Source: CAD feature listing. Evaluate the final solid. Frame: model axes, mm. Face numbers are marked on the shaded views. A direction names the side the tool comes from. Give positions to 0.01 mm unless a question says otherwise; leave off trailing zeros. Order: outer loops, then holes, each group sorted by start corner. A loop starts at its lowest first (then second) coordinate and runs counter-clockwise, first axis right, second up. Notation, with made-up numbers: (-6, -7.75) - (18, -7.75) arc R23 ccw to (18, 16.25) - close; hole circle Ø10 at (-17.75, 24.25). An arc over 180 degrees is marked (long way). Use CSV: the item, a comma, the result in double quotes.
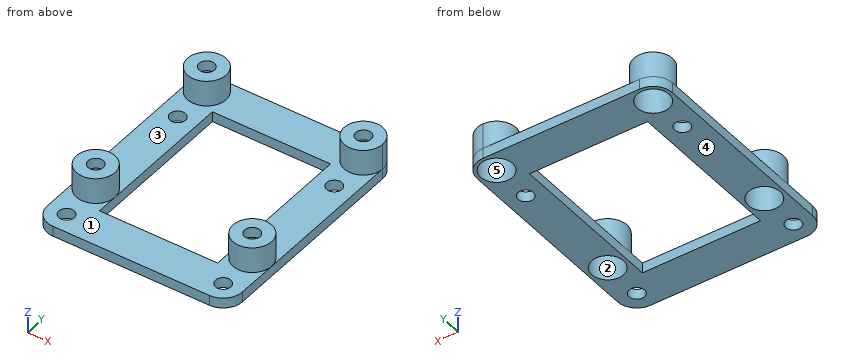
```python
from build123d import *

# Parameters (mm, degrees)
F3_W     = 38
F3_H     = 46
F3_R     = 1.5
F3_W_2   = 23
F3_H_2   = 31
F4_DEPTH = 2
F5_R     = 1.5
F6_DEPTH = 5
F7_R     = 3.7499
F8_R     = 3.1
F9_DEPTH = 5


# Not quite as in the source:
# - a fillet or chamfer is up to 0.001 mm smaller than in the source, because OpenCascade refuses the exact size


with BuildPart() as f4:
    # F3 (on Top) → F4 (new body)
    with BuildSketch(Plane.XY):
        Rectangle(F3_W, F3_H)
        with Locations((-15.25, -19.25)):
            Circle(F3_R, mode=Mode.SUBTRACT)
        with Locations((-15.25, -11.25)):
            Circle(F3_R, mode=Mode.SUBTRACT)
        with Locations((15.25, -19.25)):
            Circle(F3_R, mode=Mode.SUBTRACT)
        with Locations((15.25, -11.25)):
            Circle(F3_R, mode=Mode.SUBTRACT)
        with Locations((-15.25, 11.25)):
            Circle(F3_R, mode=Mode.SUBTRACT)
        with Locations((-15.25, 19.25)):
            Circle(F3_R, mode=Mode.SUBTRACT)
        Rectangle(F3_W_2, F3_H_2, mode=Mode.SUBTRACT)
        with Locations((15.25, 11.25)):
            Circle(F3_R, mode=Mode.SUBTRACT)
        with Locations((15.25, 19.25)):
            Circle(F3_R, mode=Mode.SUBTRACT)
    extrude(amount=F4_DEPTH)

    # F5 (on face) → F6 (join)
    with BuildSketch(Plane.XY.offset(2)):
        with BuildLine():
            ThreePointArc((-19, 19.25), (-15.25, 15.5), (-11.5, 19.25))
            ThreePointArc((-11.5, 19.25), (-12.598349559, 21.9016504179), (-15.2499999673, 23))
            ThreePointArc((-15.2499999673, 23), (-17.9016504179, 21.901650441), (-19, 19.25))
        make_face()
        with Locations((-15.25, 19.25)):
            Circle(F5_R, mode=Mode.SUBTRACT)
        with BuildLine():
            ThreePointArc((19, 19.25), (17.9016504294, 21.9016504294), (15.25, 23))
            ThreePointArc((15.25, 23), (12.5983495706, 16.5983495706), (19, 19.25))
        make_face()
        with Locations((15.25, 19.25)):
            Circle(F5_R, mode=Mode.SUBTRACT)
        with BuildLine():
            ThreePointArc((11.5, -11.25), (15.25, -15), (19, -11.25))
            ThreePointArc((19, -11.25), (15.25, -7.5), (11.5, -11.25))
        make_face()
        with Locations((15.25, -11.25)):
            Circle(F5_R, mode=Mode.SUBTRACT)
        with BuildLine():
            ThreePointArc((-11.5, -11.25), (-15.2499999923, -7.5), (-19, -11.2499999846))
            ThreePointArc((-19, -11.2499999846), (-15.2500000077, -15), (-11.5, -11.25))
        make_face()
        with Locations((-15.25, -11.25)):
            Circle(F5_R, mode=Mode.SUBTRACT)
    extrude(amount=F6_DEPTH)

    # F7 (radius 3.75 in the source; OpenCascade refuses exactly that, so slightly less here)
    f7_edges = [f4.edges().sort_by_distance(p)[0] for p in [
        (-19, 23, 1),
        (-19, -23, 1),
        (19, -23, 1),
        (19, 23, 1),
    ]]
    fillet(f7_edges, radius=F7_R)

    # F8 (on face) → F9 (cut)
    with BuildSketch(Plane(origin=(0, 0, 0), x_dir=(1, 0, 0), z_dir=(0, 0, -1))):
        with Locations((-15.25, 11.25)):
            Circle(F8_R)
        with Locations((15.25, 11.25)):
            Circle(F8_R)
        with Locations((15.25, -19.25)):
            Circle(F8_R)
        with Locations((-15.25, -19.25)):
            Circle(F8_R)
    extrude(amount=-F9_DEPTH, mode=Mode.SUBTRACT)


solid = f4.part
```
Item 1: Section A-A on y = 11.25. Return the cut outline in (x, z), then the cut area to 3 significant figures.
Filled in:
outline,"(-19, 0) - (-16.75, 0) - (-16.75, 2) - (-19, 2) - close; (-13.75, 0) - (-11.5, 0) - (-11.5, 2) - (-13.75, 2) - close; (11.5, 0) - (13.75, 0) - (13.75, 2) - (11.5, 2) - close; (16.75, 0) - (19, 0) - (19, 2) - (16.75, 2) - close"
area,"18.0 mm2"
Item 2: Mould query, pull axis Y, two halves, no side actions, for the marked faces 1 and 2. Classes: released by +Y, released by -Y, zero draft, split by the parting line, or undercut.
Filled in:
face 1,"zero draft"
face 2,"undercut"
Item 3: First-contact query: pin 1 (5 mm diameter, centred on x = -15.25, y = -11.25, fed in from -Z). Flat tip, straight axial feed; report the tip coordinate or a pass-through.
Filled in:
pin 1,"stops at z = 5"
Item 4: Material intervals for line 1 (Y direction, x = 15.25, z = 6); line 2 (X direction, y = 19.25, z = 6.3); line 3 (Y direction, x = 15.25, z = 3.7), sorted ascending. Write a range as from..to.
Filled in:
line 1,"y = -15..-12.75, -9.75..-7.5, 15.5..17.75, 20.75..23"
line 2,"x = -19..-16.75, -13.75..-11.5, 11.5..13.75, 16.75..19"
line 3,"y = -15..-14.35, -8.15..-7.5, 15.5..16.15, 22.35..23"
Item 5: Section D-D on x = 6. Return the cut outline in (y, z).
Filled in:
outline,"(-23, 0) - (-15.5, 0) - (-15.5, 2) - (-23, 2) - close; (15.5, 0) - (23, 0) - (23, 2) - (15.5, 2) - close"
Item 6: Section C-C on y = 1. Return the cut outline in (x, z).
Filled in:
outline,"(-19, 0) - (-11.5, 0) - (-11.5, 2) - (-19, 2) - close; (11.5, 0) - (19, 0) - (19, 2) - (11.5, 2) - close"
Item 7: Set-up query: the marked faces 3, 4 and 5. Return all of +Z, -Z, +X, -X, +Y, -Y with unobstructed straight access to the full face (end or side cutting, diameter ignored); none if empty.
Filled in:
face 3,"+Z"
face 4,"-Z, +X, -X, +Y, -Y"
face 5,"-Z"
Item 8: Section B-B on z = 4. Return the cut outline in (x, y).
Filled in:
outline,"circle Ø7.5 at (-15.25, -11.25); circle Ø7.5 at (-15.25, 19.25); circle Ø7.5 at (15.25, -11.25); circle Ø7.5 at (15.25, 19.25); hole circle Ø6.2 at (-15.25, -11.25); hole circle Ø6.2 at (-15.25, 19.25); hole circle Ø6.2 at (15.25, -11.25); hole circle Ø6.2 at (15.25, 19.25)"
